from build123d import *
from build123d.topology import SkipClean

# Parameters (mm, degrees)
EXTRUDE_1_DEPTH          = 15
SKETCH_2_R               = 14
EXTRUDE_2_DEPTH          = 16.5
FILLET_1_R               = 2
EXTRUDE_3_DEPTH          = 17
EXTRUDE_START            = 63
EXTRUDE_4_DEPTH          = 63
M14X1_5_1_D              = 12.5
HOLE_WIZARD_M8_1_REACH   = 67.854
HOLE_WIZARD_M8_1_BORE_R  = 3.4
CUT_EXTRUDE_1_REACH      = 67.854
CUT_EXTRUDE_1_END_RADIUS = 6.25
SKETCH_9_R               = 4.5
HOLE_WIZARD_M8_2_D       = 6.8
PATTERN_CIRCULAR_1_COUNT = 4


with BuildPart() as part:
    # 草图1 → 凸台-拉伸1 (new body)
    with BuildSketch(Plane(origin=(0, 0, 0), x_dir=(1, 0, 0), z_dir=(0, 1, 0))):
        with BuildLine():
            Line((-23.5, 31.5), (23.5, 31.5))
            ThreePointArc((23.5, 31.5), (29.156854249, 29.156854249), (31.5, 23.5))
            Line((31.5, 23.5), (31.5, -23.5))
            ThreePointArc((31.5, -23.5), (29.156854249, -29.156854249), (23.5, -31.5))
            Line((23.5, -31.5), (-23.5, -31.5))
            ThreePointArc((-23.5, -31.5), (-29.156854249, -29.156854249), (-31.5, -23.5))
            Line((-31.5, -23.5), (-31.5, 23.5))
            ThreePointArc((-31.5, 23.5), (-29.156854249, 29.156854249), (-23.5, 31.5))
        make_face()
    extrude(amount=EXTRUDE_1_DEPTH)

    # 草图2 → 凸台-拉伸2 (add)
    with BuildSketch(Plane(origin=(0, 15, 0), x_dir=(1, 0, 0), z_dir=(0, 1, 0))):
        with Locations(Location((0, 0, 0), (0, 0, 270))):
            Circle(SKETCH_2_R)
    extrude(amount=EXTRUDE_2_DEPTH)

    # 圆角1
    fillet_1_edges = [part.edges().sort_by_distance(p)[0] for p in [
        (29.156854249, 15, 29.156854249),
        (31.5, 15, 0),
        (29.156854249, 15, -29.156854249),
        (0, 15, -31.5),
        (0, 31.5, -14),
        (-29.156854249, 15, -29.156854249),
        (-31.5, 15, 0),
        (-29.156854249, 15, 29.156854249),
        (0, 15, 31.5),
    ]]
    fillet(fillet_1_edges, radius=FILLET_1_R)

    # 草图3 → 凸台-拉伸3 (add)
    with BuildSketch(Plane(origin=(0, 0, -31.5), x_dir=(-1, 0, 0), z_dir=(0, 0, -1))):
        with BuildLine():
            Line((-6.304760106, 0), (6.304760106, 0))
            ThreePointArc((6.304760106, 0), (0, 26.5), (-6.304760106, 0))
        make_face()
    extrude(amount=EXTRUDE_3_DEPTH)

    # 草图4 → 凸台-拉伸4 (add)
    with SkipClean():  # the faces are left unmerged after this step: merging them gives an invalid solid
        with BuildSketch(Plane.XY.offset(-31.5).offset(EXTRUDE_START)):
            with BuildLine():
                Line((-13.99106858, 13), (13.99106858, 13))
                ThreePointArc((13.99106858, 13), (0, 26.5), (-13.99106858, 13))
            make_face()
        extrude(amount=-EXTRUDE_4_DEPTH)

    # M14x1.5 螺纹孔1 (through all)
    with Locations(Plane(origin=(0, 0, -48.5), x_dir=(-1, 0, 0), z_dir=(0, 0, -1))):
        with Locations((0, 12.5)):
            Hole(M14X1_5_1_D / 2)

    # M8 螺纹孔1 bore → M8 螺纹孔1 (cut, up to next)
    with BuildSketch(Plane(origin=(0, 31.5, 0), x_dir=(1, 0, 0), z_dir=(0, 1, 0)), mode=Mode.PRIVATE) as hole_wizard_m8_1_sk1:
        Circle(HOLE_WIZARD_M8_1_BORE_R)
    hole_wizard_m8_1_tool1 = extrude(hole_wizard_m8_1_sk1.sketch, amount=-HOLE_WIZARD_M8_1_REACH, mode=Mode.PRIVATE) & part.part
    add(hole_wizard_m8_1_tool1.solids().sort_by_distance((0, 31.5, 0))[0], mode=Mode.SUBTRACT)

    # 切除-拉伸1: up to this cylinder (the profile starts outside it)
    with SkipClean():  # the faces are left unmerged after this step: merging them gives an invalid solid
        cut_extrude_1_end = Plane(origin=(0, 12.5, -15.5), z_dir=(0, 0, -1)) * Cylinder(CUT_EXTRUDE_1_END_RADIUS, 149.208, mode=Mode.PRIVATE)
        # 草图9 → 切除-拉伸1 (cut, up to the surface)
        with BuildSketch(Plane.XZ, mode=Mode.PRIVATE) as cut_extrude_1_sk1:
            with Locations(Location((0, -15.5, 0), (0, 0, 270))):
                Circle(SKETCH_9_R)
        cut_extrude_1_tool1 = extrude(cut_extrude_1_sk1.sketch, amount=-CUT_EXTRUDE_1_REACH, mode=Mode.PRIVATE) - cut_extrude_1_end
        add(cut_extrude_1_tool1.solids().sort_by_distance((0, 0, -15.5))[0], mode=Mode.SUBTRACT)

    # M8 螺纹孔2 (through all)
    with Locations(Plane(origin=(0, 15, 0), x_dir=(1, 0, 0), z_dir=(0, 1, 0))):
        with Locations((-22.5, 22.5)):
            hole_wizard_m8_2 = Hole(HOLE_WIZARD_M8_2_D / 2)

    # 阵列(圆周)1: M8 螺纹孔2 ×4 about axis
    with SkipClean():  # the faces are left unmerged after this step: merging them gives an invalid solid
        pattern_circular_1_axis = Axis((0, 0, 0), (0, 1, 0))
        for i in range(1, PATTERN_CIRCULAR_1_COUNT):
            add(hole_wizard_m8_2.rotate(pattern_circular_1_axis, i * 360 / PATTERN_CIRCULAR_1_COUNT), mode=Mode.SUBTRACT)


solid = part.part
Model file for the job. Use its own axes, mm. A direction names the side the tool comes from. Give positions to 0.01 mm unless a question says otherwise; leave off trailing zeros. Loops run counter-clockwise (first coordinate to the right, second up) from the corner with the lowest first, then second, coordinate; pieces in that order, holes last.
1) Flat gauge pins, fed straight in: pin 1 Ø4 at (x, z) = (0, 0) entering from +Y; pin 2 Ø4 at (x, z) = (13.5, -31.5) entering from +Y; pin 3 Ø12.5 at (x, z) = (-21.5, -14.5) entering from +Y. Where does each tip first touch, or does it go through?
2) Pull direction X, two halves, no side cores. Call faces 4 (the flat face through (6.4, 13.4, -48.5)), 5 (the cylindrical face through (-0.8, 18.7, -7.9)), 6 (the cylindrical face through (9.46, 23.76, -10.32)): +X half, -X half, draft (parallel to the pull), parting line (faces both ways), or undercut.
3) Wall check: line 1 (Z direction, x = -22.5, y = 5.5); line 2 (X direction, y = 3, z = -24). Give the ranges that are in metal, low to high.
4) Saw through at C-C (x = 0). Write the cut outline in (y, z), plus the area to 3 significant figures.
5) Saw through at B-B (x = -22.5). Write the cut outline in (y, z), plus the area to 3 significant figures.
6) Saw through at A-A (z = 22.5). Write the cut outline in (x, y), plus the area to 3 significant figures.
7) Saw through at D-D (y = 11). Write the cut outline in (x, z), plus the area to 3 significant figures.
8) Tool access for faces 1 (the cylindrical face through (-2.7, 4, -11.9)), 2 (the cylindrical face through (-18.71, 14.43, 30.9)), 3 (the flat face through (17, 6, -31.5)): list every direction of +Z, -Z, +X, -X, +Y, -Y with a clear straight run to the whole face (end or side of a thin tool).
Answer block:
1. pin 1: stops at y = 6.58
1. pin 2: stops at y = 20.48
1. pin 3: stops at y = 15
2. face 4: draft
2. face 5: undercut
2. face 6: parting line
3. line 1: z = -31.5 to -25.9, -19.1 to 19.1, 25.9 to 31.5
3. line 2: x = -31.48 to -25.55, -19.45 to 19.45, 25.55 to 31.48
4. outline: (0, -48.5) - (6.25, -48.5) - (6.25, -20) - (0, -20) - close; (0, -11) - (6.25, -11) - (6.25, 31.5) - (0, 31.5) - close; (18.75, -48.5) - (26.5, -48.5) - (26.5, -14) - (29.5, -14) arc R2 ccw to (31.5, -12) - (31.5, -3.4) - (18.75, -3.4) - close; (18.75, 3.4) - (31.5, 3.4) - (31.5, 12) arc R2 ccw to (29.5, 14) - (26.5, 14) - (26.5, 31.5) - (18.75, 31.5) - close
4. area: 1,120 mm2
5. outline: (0, -31.5) - (13, -31.5) arc R2 ccw to (15, -29.5) - (15, -25.9) - (0, -25.9) - close; (0, -19.1) - (15, -19.1) - (15, 19.1) - (0, 19.1) - close; (0, 25.9) - (15, 25.9) - (15, 29.5) arc R2 ccw to (13, 31.5) - (0, 31.5) - close
5. area: 739 mm2
6. outline: (-31.5, 0) - (-25.9, 0) - (-25.9, 15) - (-29.5, 15) arc R2 ccw to (-31.5, 13) - close; (-19.1, 0) - (19.1, 0) - (19.1, 15) - (13.77, 15) arc R14 ccw to (-13.77, 15) - (-19.1, 15) - close; (25.9, 0) - (31.5, 0) - (31.5, 13) arc R2 ccw to (29.5, 15) - (25.9, 15) - close; hole circle Ø12.5 at (0, 12.5)
6. area: 855 mm2
7. outline: (-31.5, -23.5) arc R8 ccw to (-23.5, -31.5) - (-13.92, -31.5) - (-13.92, -48.5) - (-6.07, -48.5) - (-6.07, 31.5) - (-23.5, 31.5) arc R8 ccw to (-31.5, 23.5) - close; (6.07, -48.5) - (13.92, -48.5) - (13.92, -31.5) - (23.5, -31.5) arc R8 ccw to (31.5, -23.5) - (31.5, 23.5) arc R8 ccw to (23.5, 31.5) - (6.07, 31.5) - close; hole circle Ø6.8 at (-22.5, -22.5); hole circle Ø6.8 at (-22.5, 22.5); hole circle Ø6.8 at (22.5, -22.5); hole circle Ø6.8 at (22.5, 22.5)
7. area: 3,270 mm2
8. face 1: -Y
8. face 2: +Z, -X, +Y
8. face 3: -Z, +X, -Y
